Part model, mm, in its own coordinate system. A direction names the side the tool comes from. Give positions to 0.01 mm unless a question says otherwise; leave off trailing zeros. Write each loop counter-clockwise with the first axis right and the second up, starting at its lowest first coordinate (ties: lowest second). Pieces come first, ordered by that corner, then holes. Notation, with made-up numbers: M -11,-12.75 L 31,-12.75 A18 cw 31,3.25 Z; hole C 40,49.25 d5. An arc over 180 degrees is marked long. Use CSV: the item, a comma, the result in double quotes. Start each with the question number.
1. Band-saw the part on A-A, the plane x = 0. List the corners of the cut face in (y, z).
2. Drill centre lines: line 1 along Z through (x, y) = (0, 5); line 2 along X through (y, z) = (5, 56); line 3 along X through (y, z) = (3.5, 56). Where is each one in solid material? Low to high. Write a range as from..to.
3. Drop flat-ended pins along their axis: pin 1 Ø1 at (y, z) = (6, 54.5) entering from -X; pin 2 Ø1.5 at (x, z) = (3.5, 49.5) entering from -Y; pin 3 Ø6 at (x, z) = (8.5, 46) entering from -Y; pin 4 Ø5 at (x, z) = (0, 56) entering from -Y. Give the stop position or say it passes through.
4. Mould opens along X. For faces 3 (the face through (0.1, -13.4, 42)), 4 (the face through (-8.06, -12.65, 20.71)), 5 (the face through (-1.532, -0.182, 59.695)) say: pulls with the +X half, pulls with the -X half, needs draft (parallel to the pull), parting line crosses it, or undercut.
5. Band-saw the part on C-C, the plane z = 56. List the corners of the cut face in (x, y), then the cut area to 3 significant figures.
6. Band-saw the part on B-B, the plane y = 0. List the corners of the cut face in (x, z).
7. 3-axis set-ups, long thin cutter, end or side, ignore diameter. For faces 1 (the face through (0, 0, 67)), 2 (the face through (12.4, 3.9, 53.3)): which of +Z, -Z, +X, -X, +Y, -Y reach the whole face in a straight line?
8. Band-saw the part on D-D, the plane z = 23.5. List the corners of the cut face in (x, y), then the cut area to 3 significant figures.
from build123d import *

# Parameters (mm, degrees)
SCHIZZO1_R             = 15
ESTRUSIONE1_DEPTH      = 42
SCHIZZO2_R             = 13
ESTRUSIONE2_DEPTH      = 25
SMUSSO1_SIZE           = 2
ESTRUSIONE3_DEPTH      = 71.278019323
ESTRUSIONE3_DEPTH_BACK = 71.278019323
SCHIZZO3_R             = 4


with BuildPart() as part:
    # Schizzo1 → Estrusione1 (new body)
    with BuildSketch(Plane.XY):
        with Locations(Location((0, 0, 0), (0, 0, 180))):
            Circle(SCHIZZO1_R)
    extrude(amount=ESTRUSIONE1_DEPTH)

    # Schizzo2 → Estrusione2 (add)
    with BuildSketch(Plane.XY.offset(42)):
        Circle(SCHIZZO2_R)
    extrude(amount=ESTRUSIONE2_DEPTH)

    # Smusso1
    smusso1_edges = [part.edges().sort_by_distance(p)[0] for p in [
        (-13, 0, 67),
    ]]
    chamfer(smusso1_edges, length=SMUSSO1_SIZE)

    # Schizzo3 → Estrusione3 (cut, two sides: drawn at the far end of the back side and taken through both)
    with BuildSketch(Plane(origin=(0, 0, 0), x_dir=(1, 0, 0), z_dir=(0, 1, 0)).offset(-ESTRUSIONE3_DEPTH_BACK)):
        with Locations(Location((0, -56, 0), (0, 0, 270))):
            Circle(SCHIZZO3_R)
    extrude(amount=ESTRUSIONE3_DEPTH + ESTRUSIONE3_DEPTH_BACK, mode=Mode.SUBTRACT)


solid = part.part
Output:
1,outline,"M -15,0 L 15,0 L 15,42 L 13,42 L 13,52 L -13,52 L -13,42 L -15,42 Z; M -13,60 L 13,60 L 13,65 L 11,67 L -11,67 L -13,65 Z"
2,line 1,"z = 0..52, 60..67"
2,line 2,"x = -12..-4, 4..12"
2,line 3,"x = -12.52..-4, 4..12.52"
3,pin 1,"stops at x = -11.78"
3,pin 2,"stops at y = -12.71"
3,pin 3,"stops at y = -11.78"
3,pin 4,"passes through"
4,face 3,"needs draft"
4,face 4,"parting line crosses it"
4,face 5,"undercut"
5,outline,"M -4,-12.37 L -4,12.37 A13 ccw Z; M 4,-12.37 A13 ccw 4,12.37 Z"
5,area,"326 mm²"
6,outline,"M -15,0 L 15,0 L 15,42 L 13,42 L 13,65 L 11,67 L -11,67 L -13,65 L -13,42 L -15,42 Z; hole C 0,56 d8"
7,face 1,"+Z, +X, -X, +Y, -Y"
7,face 2,"+Z"
8,outline,"C 0,0 d30"
8,area,"707 mm²"
